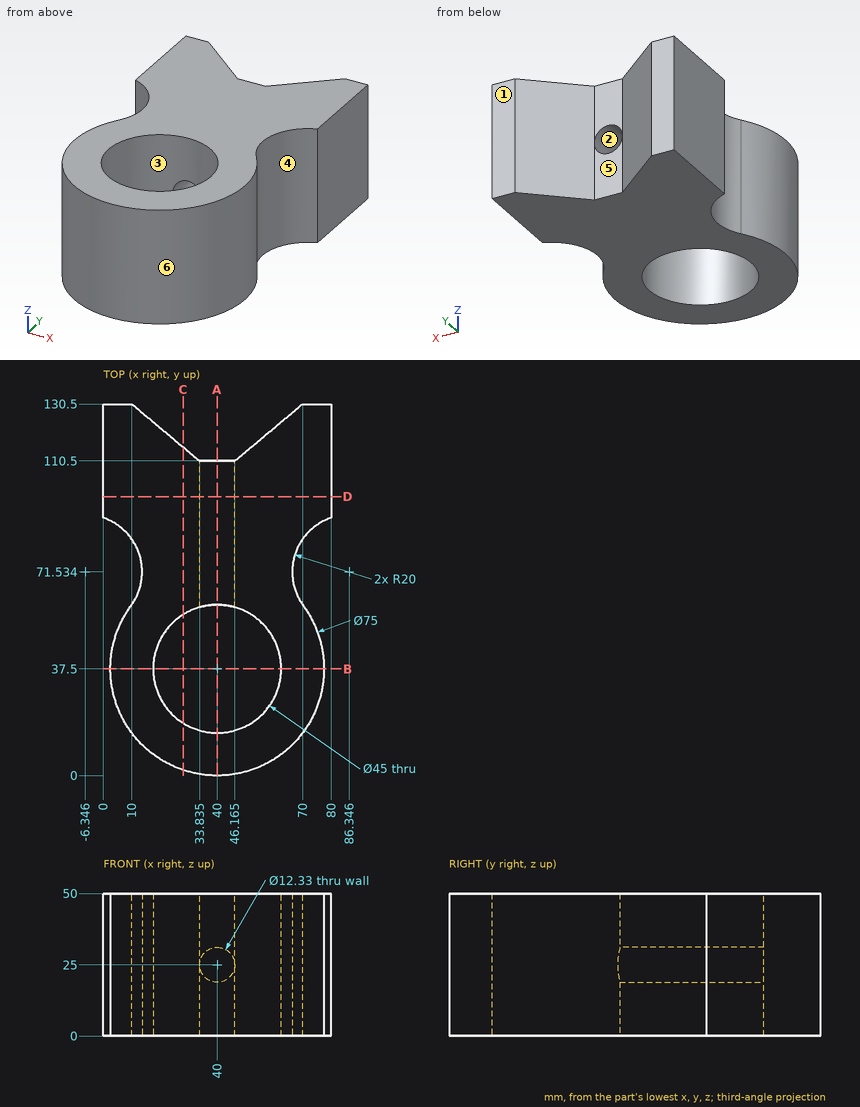
Geometry: see drawing. Coordinates: mm, zero at the bounding-box minimum. A direction names the side the tool comes from. Coordinates: 2 decimals unless noted, no trailing zeros. Write each loop counter-clockwise with the first axis right and the second up, starting at its lowest first coordinate (ties: lowest second). Pieces come first, ordered by that corner, then holes.
1) Section C-C on x = 28. Output: boundary loops of the cut face in (y, z).
2) Section A-A on x = 40. Output: boundary loops of the cut face in (y, z) (1 decimal).
3) Material intervals for line 1 along Z through (x, y) = (40, 78) (1 decimal); line 2 along X through (y, z) = (98, 25) (1 decimal); line 3 along Y through (x, z) = (40, 33), sorted ascending.
4) Section D-D on y = 98. Output: boundary loops of the cut face in (x, z) (1 decimal).
5) Section B-B on y = 37.5. Output: boundary loops of the cut face in (x, z).
6) Set-up query: the marked faces 5 and 6. Return all of +Z, -Z, +X, -X, +Y, -Y with unobstructed straight access to the full face (end or side cutting, diameter ignored); none if empty.
7) Pin query (flat end, axial travel): pin 1 Ø6 at (y, z) = (30.5, 31) entering from -X; pin 2 Ø8 at (y, z) = (69.5, 36) entering from +X; pin 3 Ø19.5 at (x, z) = (40, 25) entering from +Y. Return the tip coordinate at first contact, or that it passes through.
8) Mould query, pull axis Y, two halves, no side actions, for the marked faces 1, 2, 3 and 4. Classes: pulls with the +Y half, pulls with the -Y half, needs draft (parallel to the pull), parting line crosses it, or undercut.
Check result:
1. outline: (1.97, 0) - (18.47, 0) - (18.47, 50) - (1.97, 50) - close; (56.53, 0) - (115.4, 0) - (115.4, 50) - (56.53, 50) - close
2. outline: (0, 0) - (15, 0) - (15, 50) - (0, 50) - close; (60, 0) - (110.5, 0) - (110.5, 18.8) - (60, 18.8) - close; (60, 31.2) - (110.5, 31.2) - (110.5, 50) - (60, 50) - close
3. line 1: z = 0 to 18.8, 31.2 to 50
3. line 2: x = 0 to 33.8, 46.2 to 80
3. line 3: y = 0 to 15, 60 to 110.5
4. outline: (0, 0) - (80, 0) - (80, 50) - (0, 50) - close; hole circle Ø12.3 at (40, 25)
5. outline: (2.5, 0) - (17.5, 0) - (17.5, 50) - (2.5, 50) - close; (62.5, 0) - (77.5, 0) - (77.5, 50) - (62.5, 50) - close
6. face 5: +Z, -Z, +Y
6. face 6: +Z, -Z
7. pin 1: stops at x = 2.71
7. pin 2: stops at x = 67.28
7. pin 3: stops at y = 113.51
8. face 1: pulls with the +Y half
8. face 2: needs draft
8. face 3: undercut
8. face 4: undercut
